Verification items for the finished model (mm, model axes). Give positions to 0.01 mm unless a question says otherwise; leave off trailing zeros. Order: outer loops, then holes, each group sorted by start corner. A loop starts at its lowest first (then second) coordinate and runs counter-clockwise, first axis right, second up. Notation, with made-up numbers: (20, -39.75) -> (52, -39.75) arc R30 cw to (52, -8.75) -> close; hole circle Ø11 at (15.5, 63.25). An arc over 180 degrees is marked (long way). Write each question's results on one line, items separated by ' | '. Start each with the question number.
1. Cross-section at C-C, the plane z = -4.5. Enter the section's corners in (x, y), then the cut area to 4 significant figures.
2. Cross-section at A-A, the plane z = -14.5. Enter the section's corners in (x, y), then the cut area to 3 significant figures.
3. Material ranges on L1, parallel to X at y = 0.1, z = -14.5; L2, parallel to X at y = 0.2, z = -1.75; L3, parallel to X at y = 0.2, z = -15, recorded low to high. Write a range as from..to.
4. Cross-section at B-B, the plane y = 0.25. Enter the section's corners in (x, z).
5. Depth check by flat-ended pin: pin 1 Ø4 at (x, z) = (0.5, -23) entering from -Y. Enter the tip coordinate at first touch or a pass-through.
Autodesk Inventor part; units mm, degrees
ref_plane "YZ Plane" through (0, 0, 0) normal (1, 0, 0) x (0, 1, 0)
ref_plane "XZ Plane" through (0, 0, 0) normal (0, 1, 0) x (-1, 0, 0)
ref_plane "XY Plane" through (0, 0, 0) normal (0, 0, 1) x (1, 0, 0)
sketch "Sketch1" plane through (0, 0, 0) normal (0, 1, 0) x (-1, 0, 0)
  line L0 (0, 0) -> (-9.5, 0)
  line L1 (-9.5, 0) -> (-9.5, -29)
  line L2 (-9.5, -29) -> (0, -29)
  line L3 (0, -29) -> (0, 0)
  dimension "d0" = 9.5
  dimension "d1" = 29
extrude "Extrusion1" add sketch "Sketch1" along normal blind 0.5
sketch "Sketch3" plane through (0, 0.5, 0) normal (0, 1, 0) x (1, 0, 0)
  circle A0 centre (9.5, 24.5) radius 0.75
  circle A1 centre (9.5, 24.5) radius 0.5
  circle A2 centre (9.5, 4.5) radius 0.75
  circle A3 centre (9.5, 4.5) radius 0.5
  point P0 (0, 0)
  point P1 (9.5, 0)
  point P2 (9.5, 29)
  dimension "d6" = 1.5
  dimension "d7" = 1
  dimension "d8" = 1.5
  dimension "d9" = 1
extrude "Extrusion2" add sketch "Sketch3" against normal blind 0.5
sketch "Sketch4" plane through (0, 0.5, 0) normal (0, 1, 0) x (1, 0, 0)
  line L0 (0, 29) -> (0, 0)
  line L1 (0, 29) -> (0, 14.5)
  circle A0 centre (0, 14.5) radius 1.25
  circle A1 centre (0, 14.5) radius 0.75
  point P0 (0, 13.75)
  point P1 (0, 15.25)
  point P2 (0, 15.75)
  point P3 (0, 13.25)
  dimension "d12" = 14.5
  dimension "d13" = 2.5
  dimension "d14" = 1.5
extrude "Extrusion3" add sketch "Sketch4" against normal blind 0.5 contours L0 A1 A0 picked at (-1.0514, 14.2719)
properties part number "Shelf"
Results below:
1) outline: (0, 0) -> (9.5, 0) -> (9.5, 0.5) -> (0, 0.5) -> close; (10, 0) -> (10.25, 0) -> (10.25, 0.5) -> (10, 0.5) -> close | area: 4.875 mm²
2) outline: (-1.25, 0) -> (-0.75, 0) -> (-0.75, 0.5) -> (-1.25, 0.5) -> close; (0, 0) -> (9.5, 0) -> (9.5, 0.5) -> (0, 0.5) -> close | area: 5.00 mm²
3) L1: x = -1.25..-0.75, 0..9.5 | L2: x = 0..9.5 | L3: x = -1.15..-0.56, 0..9.5
4) outline: (0, -29) -> (9.5, -29) -> (9.5, -25.25) arc R0.75 ccw to (9.5, -23.75) -> (9.5, -5.25) arc R0.75 ccw to (9.5, -3.75) -> (9.5, 0) -> (0, 0) -> (0, -13.25) arc R1.25 ccw to (0, -15.75) -> close; hole (0, -15.25) -> (0, -13.75) arc R0.75 ccw to start; hole (9.5, -25) arc R0.5 ccw to (9.5, -24) -> close; hole (9.5, -5) arc R0.5 ccw to (9.5, -4) -> close
5) pin 1: stops at y = 0
